```python
from build123d import *

# Parameters (mm, degrees)
BOSS_EXTRUDE1_DEPTH = 3.175
SKETCH3_R           = 2.38125
CUT_EXTRUDE1_DEPTH  = 439.000935786


with BuildPart() as part:
    # Sketch2 → Boss-Extrude1 (new body)
    with BuildSketch(Plane.XY):
        Polygon((50.8, 0), (381, 190.641058886), (381, 216.041058886), (330.2, 216.041058886), (50.8, 50.8), (0, 50.8), (0, 0), align=None)
    extrude(amount=BOSS_EXTRUDE1_DEPTH)

    # Sketch3 → Cut-Extrude1 (cut, through all)
    with BuildSketch(Plane.XY.offset(3.175)):
        with Locations((12.7, 12.7)):
            Circle(SKETCH3_R)
        with Locations((12.7, 38.1)):
            Circle(SKETCH3_R)
        with Locations(Location((342.9, 203.341058886, 0), (0, 0, 180))):
            Circle(SKETCH3_R)
        with Locations(Location((368.3, 203.341058886, 0), (0, 0, 180))):
            Circle(SKETCH3_R)
        with Locations((38.1, 12.7)):
            Circle(SKETCH3_R)
        with Locations((38.1, 38.1)):
            Circle(SKETCH3_R)
    extrude(amount=-CUT_EXTRUDE1_DEPTH, mode=Mode.SUBTRACT)


solid = part.part
```
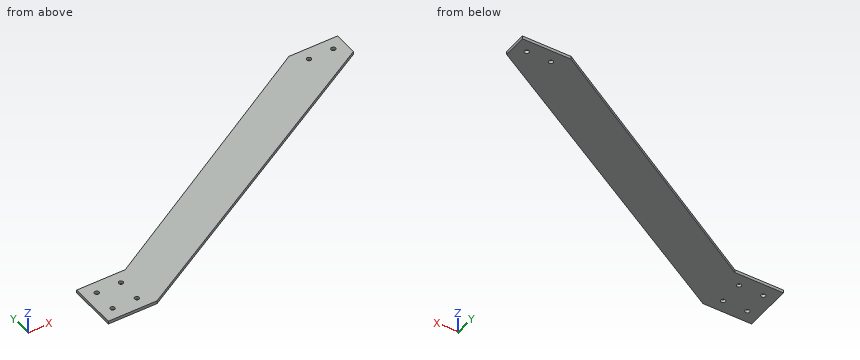
Check sheet for the modelled part. Datum: model origin and axes. Units: mm. Coordinates: 2 decimals unless noted, no trailing zeros. Loops run counter-clockwise (first coordinate to the right, second up) from the corner with the lowest first, then second, coordinate; pieces in that order, holes last. Notation, with made-up numbers: M -8.75,-1 L 9.25,-1 A34 ccw 9.25,30 Z; hole C 87.25,12.5 d7. An arc over 180 degrees is marked long. Answer as a JSON object with one key per item and string values.
1. Depth check by flat-ended pin: P1, Ø1.5, axis at x = 160.5, z = 2.5, coming from the -Y side. Enter the tip coordinate at first touch or a pass-through.
Outcome:
{"P1": "y = 62.9"}
2. Sectioned sample at A-A on z = 2.25. Record the cut outline in (x, y), and give its area (3 significant figures).
Outcome:
{"outline": "M 0,0 L 50.8,0 L 381,190.64 L 381,216.04 L 330.2,216.04 L 50.8,50.8 L 0,50.8 Z; hole C 12.7,12.7 d4.76; hole C 12.7,38.1 d4.76; hole C 38.1,12.7 d4.76; hole C 38.1,38.1 d4.76; hole C 342.9,203.34 d4.76; hole C 368.3,203.34 d4.76", "area": "19,300 mm²"}
3. Sectioned sample at C-C on y = 30. Record the cut outline in (x, z) (3 decimals).
Outcome:
{"outline": "M 0,0 L 102.762,0 L 102.762,3.175 L 0,3.175 Z"}
4. Sectioned sample at B-B on x = 28.5. Record the cut outline in (y, z) (3 decimals), and give its area (3 significant figures).
Outcome:
{"outline": "M 0,0 L 50.8,0 L 50.8,3.175 L 0,3.175 Z", "area": "161 mm²"}
5. Scan lines: L1, parallel to Y at x = 12.7, z = 1.3; L2, parallel to Y at x = 368.3, z = 1.6; L3, parallel to X at y = 14, z = 2.9. Record each from-to range of solid material in increasing order. Write a range as from..to.
Outcome:
{"L1": "0..10.32, 15.08..35.72, 40.48..50.8", "L2": "183.31..200.96, 205.72..216.04", "L3": "0..10.7, 14.7..36.1, 40.1..75.05"}
